```python
from build123d import *

# Parameters (mm, degrees)
BOSS_EXTRU_1_DEPTH = 10
ESQUISSE2_W        = 35
ESQUISSE2_H        = 20
BOSS_EXTRU_2_DEPTH = 10


with BuildPart() as part:
    # Esquisse1 → Boss.-Extru.1 (new body)
    with BuildSketch(Plane.XY):
        with BuildLine():
            Line((5, 65), (40, 65))
            Line((40, 65), (40, -65))
            Line((40, -65), (5, -65))
            ThreePointArc((5, -65), (-26.819805153, -51.819805153), (-40, -20))
            Line((-40, -20), (-40, 20))
            ThreePointArc((-40, 20), (-26.819805153, 51.819805153), (5, 65))
        make_face()
        with BuildLine():
            Line((0, 50), (25, 50))
            Line((25, 50), (25, -50))
            Line((25, -50), (0, -50))
            ThreePointArc((0, -50), (-17.67766953, -42.67766953), (-25, -25))
            Line((-25, -25), (-25, 25))
            ThreePointArc((-25, 25), (-17.67766953, 42.67766953), (0, 50))
        make_face(mode=Mode.SUBTRACT)
    extrude(amount=BOSS_EXTRU_1_DEPTH)

    # Esquisse2 → Boss.-Extru.2 (add)
    with BuildSketch(Plane.XY.offset(10)):
        with Locations((57.5, 30)):
            Rectangle(ESQUISSE2_W, ESQUISSE2_H)
        with Locations((57.5, -30)):
            Rectangle(ESQUISSE2_W, ESQUISSE2_H)
    extrude(amount=-BOSS_EXTRU_2_DEPTH)


solid = part.part
```
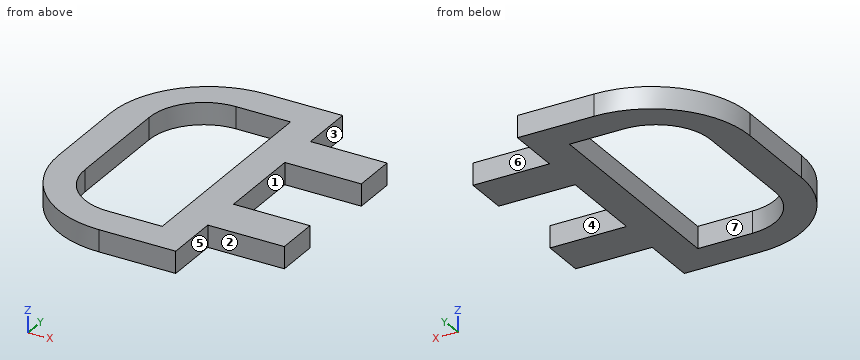
Verification items for the finished model (mm, model axes). Face numbers are marked on the shaded views. A direction names the side the tool comes from. Coordinates: 2 decimals unless noted, no trailing zeros. Write each loop counter-clockwise with the first axis right and the second up, starting at its lowest first coordinate (ties: lowest second). Pieces come first, ordered by that corner, then holes. Notation, with made-up numbers: (49, 58.25) - (53, 58.25) arc R23 cw to (53, 89.25) - close; hole circle Ø1 at (45, 6). An arc over 180 degrees is marked (long way). One line per question, with ' | ' between items. Start each with the question number.
1. Section check C-C (z = 8.5). Enter the section's corners in (x, y), plus the area to 3 significant figures.
2. Gauge pin test, flat ends, axial feed: P1, Ø6, axis at x = -1.5, z = 7, coming from the +Y side; P2, Ø5, axis at x = 60, z = 9, coming from the -Y side; P3, Ø1, axis at y = 46, z = 3, coming from the -X side. Record the tip position at first contact, or that the pin passes through.
3. Material ranges on line 1 along Y through (x, z) = (8.5, 4); line 2 along X through (y, z) = (12, 4.25); line 3 along Y through (x, z) = (60.5, 5), recorded low to high.
4. Access from +Z, -Z, +X, -X, +Y, -Y to the whole of each face (thin tool, end or side, straight path). Record for the marked faces 4, 5, 6 and 7.
5. Section check B-B (y = -14). Enter the section's corners in (x, z).
6. Draft check along Y on the marked faces 1, 2 and 3. Enter one of: released by +Y, released by -Y, zero draft, split by the parting line, or undercut.
7. Section check A-A (x = 56). Enter the section's corners in (y, z).
Computed values:
1) outline: (-40, -20) arc R45 ccw to (5, -65) - (40, -65) - (40, -40) - (75, -40) - (75, -20) - (40, -20) - (40, 20) - (75, 20) - (75, 40) - (40, 40) - (40, 65) - (5, 65) arc R45 ccw to (-40, 20) - close; hole (-25, -25) arc R25 ccw to (0, -50) - (25, -50) - (25, 50) - (0, 50) arc R25 ccw to (-25, 25) - close | area: 6,200 mm²
2) P1: y = 64.86 | P2: y = -40 | P3: x = -32.08
3) line 1: -65 to -50, 50 to 65 | line 2: -40 to -25, 25 to 40 | line 3: -40 to -20, 20 to 40
4) face 4: +Z, -Z, +X | face 5: +Z, -Z, +X, -Y | face 6: +Z, -Z, +X, +Y | face 7: +Z, -Z
5) outline: (-40, 0) - (-25, 0) - (-25, 10) - (-40, 10) - close; (25, 0) - (40, 0) - (40, 10) - (25, 10) - close
6) face 1: undercut | face 2: released by -Y | face 3: zero draft
7) outline: (-40, 0) - (-20, 0) - (-20, 10) - (-40, 10) - close; (20, 0) - (40, 0) - (40, 10) - (20, 10) - close
